Read the model definition and answer for the solid it produces. Units are mm, in the model's axes. A direction names the side the tool comes from. Coordinates: 2 decimals unless noted, no trailing zeros. Order: outer loops, then holes, each group sorted by start corner. A loop starts at its lowest first (then second) coordinate and runs counter-clockwise, first axis right, second up. Notation, with made-up numbers: (-31.75, -5.75) - (-22.75, -5.75) arc R12 ccw to (-22.75, 4.25) - close; hole circle Ø10 at (-10, -25). An arc over 180 degrees is marked (long way). Use one line per item in the form item = value.
Autodesk Inventor part; units mm, degrees
ref_plane "XZ Plane" through (0, 0, 0) normal (0, 1, 0) x (-1, 0, 0)
sketch "Sketch3" plane through (0, 0, 0) normal (0, 1, 0) x (-1, 0, 0)
  line L0 (15.24, 19.685) -> (-15.24, 19.685)
  line L1 (-15.24, 19.685) -> (-15.24, -19.685)
  line L2 (-15.24, -19.685) -> (15.24, -19.685)
  line L3 (15.24, -19.685) -> (15.24, 19.685)
  line L4 (15.24, 19.685) -> (-15.24, -19.685) construction
  line L5 (-15.24, 19.685) -> (15.24, -19.685) construction
  line L6 (-12.7, 17.145) -> (-12.7, -17.145)
  line L7 (-12.7, -17.145) -> (12.7, -17.145)
  line L8 (12.7, -17.145) -> (12.7, 17.145)
  line L9 (12.7, 17.145) -> (-12.7, 17.145)
  line L10 (-12.7, 17.145) -> (12.7, -17.145) construction
  line L11 (-12.7, -17.145) -> (12.7, 17.145) construction
  point P0 (0, 0)
  dimension "d11" = 30.48
  dimension "d12" = 39.37
  dimension "d13" = 34.29
  dimension "d14" = 25.4
extrude "Extrusion4" add sketch "Sketch3" along normal blind 18.2626
sketch "Sketch4" plane through (0, 0, 0) normal (0, -1, 0) x (1, 0, 0)
  line L0 (12.7, 17.145) -> (-12.7, 17.145)
  line L1 (-12.7, -17.145) -> (12.7, -17.145)
  line L2 (12.7, 17.145) -> (-12.7, 17.145)
  line L3 (-12.7, 17.145) -> (-12.7, -17.145)
  line L4 (-12.7, -17.145) -> (12.7, -17.145)
  line L5 (12.7, -17.145) -> (12.7, 17.145)
  point P0 (0, 0)
extrude "Extrusion5" add sketch "Sketch4" against normal blind 3.81
sketch "Sketch5" plane through (0, 3.81, 0) normal (0, 1, 0) x (1, 0, 0)
  line L0 (10.795, -15.24) -> (10.795, 15.24)
  line L1 (10.795, 15.24) -> (-10.795, 15.24)
  line L2 (-10.795, 15.24) -> (-10.795, -15.24)
  line L3 (-10.795, -15.24) -> (10.795, -15.24)
  line L4 (10.795, -15.24) -> (-10.795, 15.24) construction
  line L5 (10.795, 15.24) -> (-10.795, -15.24) construction
  line L6 (12.7, -17.145) -> (-12.7, -17.145)
  line L7 (12.7, 17.145) -> (12.7, -17.145)
  line L8 (-12.7, 17.145) -> (12.7, 17.145)
  line L9 (12.7, -17.145) -> (-12.7, -17.145)
  line L10 (-12.7, -17.145) -> (-12.7, 17.145)
  line L11 (-12.7, 17.145) -> (12.7, 17.145)
  line L12 (12.7, 17.145) -> (12.7, -17.145)
  point P0 (0, 0)
  dimension "d21" = 1.905
  dimension "d22" = 1.905
extrude "Extrusion6" add sketch "Sketch5" along normal blind 3.9878
sketch "Sketch6" plane through (0, 0, 0) normal (0, -1, 0) x (1, 0, 0)
  line L0 (15.24, 19.685) -> (15.24, -19.685) construction
  line L1 (15.24, -13.081) -> (-15.24, -13.081) construction
  line L2 (-15.24, -19.685) -> (-15.24, 19.685) construction
  line L3 (15.24, -19.685) -> (-15.24, -19.685) construction
  point P0 (0, 0)
  point P1 (8.89, -13.081)
  point P2 (-8.89, -13.081)
  dimension "d25" = 6.604
  dimension "d26" = 6.35
  dimension "d27" = 6.35
hole "Hole1" at (8.89, 0, -13.081) at (-8.89, 0, -13.081) direction (0, 1, 0) diameter 2.159 end through all
sketch "Sketch8" plane through (-15.24, 0, 19.685) normal (0, 0, 1) x (1, 0, 0)
  line L0 (15.24, 0) -> (20.32, 0)
  line L1 (20.32, 0) -> (20.32, 5.08)
  line L2 (20.32, 5.08) -> (15.24, 5.08)
  line L3 (15.24, 5.08) -> (15.24, 0)
  line L4 (15.24, 0) -> (10.16, 0)
  line L5 (10.16, 0) -> (10.16, 5.08)
  line L6 (10.16, 5.08) -> (15.24, 5.08)
  dimension "d35" = 5.08
  dimension "d36" = 5.08
extrude "Extrusion7" add sketch "Sketch8" along normal blind 12.7
sketch "Sketch10" plane through (-5.08, 5.08, 19.685) normal (0, 1, 0) x (1, 0, 0)
  line L0 (-10.16, 0) -> (20.32, 0)
  line L1 (0, 0) -> (0, -12.7)
  point P0 (5.08, 19.685)
  point P1 (5.08, -6.35)
  dimension "d46" = 6.35
  dimension "d54" = 5.08
hole "Hole3" at (0, 5.08, 26.035) direction (0, -1, 0) diameter 6.35 end through all
mirror "Mirror1" about plane through (0, 0, 0) normal (0, 0, 1) of "Hole3", "Extrusion7"
equation "\"d11\" = caseWidth"
equation "\"d12\" = caseLength"
equation "\"d13\" = internalCaseLength"
equation "\"d14\" = internalCaseWidth"
equation "\"d17\" = caseHeight"
equation "\"d19\" = caseBaseThickness"
equation "\"d21\" = supportWidth"
equation "\"d22\" = supportWidth"
equation "\"d23\" = componentHeightAboveBoard"
equation "\"d35\" = tabHeight"
equation "\"d36\" = halfTabWidth"
equation "\"d37\" = tabLength"
equation "\"boardWidth\" = 22.86"
equation "\"boardLength\" = 31.75"
equation "\"boardThickness\" = 1.7272"
equation "\"componentHeightAboveBoard\" = 3.9878"
equation "\"headerHeightAboveBard\" = 8.7376"
equation "\"holeDiam\" = 2.3368"
equation "\"centerLineForHoles\" = 2.794"
equation "\"holeDistanceFromEdge\" = 2.54"
equation "\"supportWidth\" = 1.905"
equation "\"caseWallWidth\" = 2.54"
equation "\"internalSpacingForComponent\" = 1.27"
equation "\"caseWidth\" = 2 * caseWallWidth + boardWidth + 2 * internalSpacingForComponent"
equation "\"caseLength\" = 2 * caseWallWidth + boardLength + 2 * internalSpacingForComponent"
equation "\"internalCaseWidth\" = boardWidth + 2 * internalSpacingForComponent"
equation "\"internalCaseLength\" = boardLength + 2 * internalSpacingForComponent"
equation "\"caseHeight\" = headerHeightAboveBard + boardThickness + componentHeightAboveBoard + caseBaseThickness"
equation "\"caseBaseThickness\" = 3.81"
equation "\"tabHeight\" = 5.08"
equation "\"tabWidth\" = 10.16"
equation "\"halfTabWidth\" = 0.5 * tabWidth"
equation "\"tabLength\" = 12.7"
equation "\"halfTabLength\" = 0.5 * tabLength"
properties part number "CaseForADXL_345" material "ABS Plastic"
(1) The mould has two halves that part along Z. Classify faces 5 (the flat face through (-12.7, 13, 0)), 6 (the flat face through (-5.08, 3, -26)): +Z half, -Z half, draft (parallel to the pull), parting line (faces both ways), or undercut.
Answer list:
face_5 = undercut
face_6 = draft
(2) Given pin 1 Ø3 at (x, z) = (-8.89, -13.081) entering from -Y; pin 2 Ø1.5 at (y, z) = (3, -23.5) entering from -X; pin 3 Ø3 at (x, y) = (-4.5, 14) entering from -Z (3 decimals); pin 4 Ø12 at (x, z) = (3, -6) entering from +Y, each flat-ended and moving along its own axis, determine where each tip first touches the part or whether it passes through.
Answer list:
pin_1 = 0
pin_2 = -5.08
pin_3 = -19.685
pin_4 = 3.81
(3) Straight lines are drawn through the part: L1, parallel to Z at x = 0, y = 3.2 (3 decimals); L2, parallel to Z at x = -9.5, y = 9.5 (3 decimals); L3, parallel to X at y = 9.25, z = -11. For each, find the intervals that lie inside material, in ascending order.
Answer list:
L1 = -32.385 to -29.21, -22.86 to 22.86, 29.21 to 32.385
L2 = -19.685 to -17.145, 17.145 to 19.685
L3 = -15.24 to -12.7, 12.7 to 15.24
(4) Section B-B, the plane x = -8.89 is taken. Write down the section's boundary in (y, z) (1 decimal).
Answer list:
outline = (0, -19.7) - (18.3, -19.7) - (18.3, -17.1) - (7.8, -17.1) - (7.8, -15.2) - (3.8, -15.2) - (3.8, -14.2) - (0, -14.2) - close; (0, -12) - (3.8, -12) - (3.8, 15.2) - (7.8, 15.2) - (7.8, 17.1) - (18.3, 17.1) - (18.3, 19.7) - (0, 19.7) - close
(5) Section A-A, the plane x = 0 is taken. Write down the section's boundary in (y, z) (3 decimals), then the cut area to 3 significant figures.
Answer list:
outline = (0, -32.385) - (5.08, -32.385) - (5.08, -29.21) - (0, -29.21) - close; (0, -22.86) - (5.08, -22.86) - (5.08, -19.685) - (18.263, -19.685) - (18.263, -17.145) - (7.798, -17.145) - (7.798, -15.24) - (3.81, -15.24) - (3.81, 15.24) - (7.798, 15.24) - (7.798, 17.145) - (18.263, 17.145) - (18.263, 19.685) - (5.08, 19.685) - (5.08, 22.86) - (0, 22.86) - close; (0, 29.21) - (5.08, 29.21) - (5.08, 32.385) - (0, 32.385) - close
area = 303 mm2
(6) Section D-D, the plane y = 15.25 is taken. Write down the section's boundary in (x, z) (3 decimals).
Answer list:
outline = (-15.24, -19.685) - (15.24, -19.685) - (15.24, 19.685) - (-15.24, 19.685) - close; hole (-12.7, -17.145) - (12.7, -17.145) - (12.7, 17.145) - (-12.7, 17.145) - close
(7) Section C-C, the plane z = -27.5 is taken. Write down the section's boundary in (x, y).
Answer list:
outline = (-5.08, 0) - (-2.82, 0) - (-2.82, 5.08) - (-5.08, 5.08) - close; (2.82, 0) - (5.08, 0) - (5.08, 5.08) - (2.82, 5.08) - close
(8) Which of the six approach directions +Z, -Z, +X, -X, +Y, -Y give full straight-line access (tool end or side, diameter ignored) to faces 1 (the flat face through (3.5, 5.08, 25.9)), 2 (the flat face through (-3.5, 5.08, -25.9)), 3 (the flat face through (5.08, 3, 26)), 4 (the flat face through (0, 6, 15.24))?
Answer list:
face_1 = +Z, +X, -X, +Y
face_2 = -Z, +X, -X, +Y
face_3 = +Z, +X, +Y, -Y
face_4 = +Y
